from build123d import *

# Parameters (mm, degrees)
SKETCH1_R           = 12.5
SKETCH1_R_2         = 8
BOSS_EXTRUDE1_DEPTH = 2.5
SKETCH3_R           = 20
SKETCH3_R_2         = 8
BOSS_EXTRUDE3_DEPTH = 5
CHAMFER2_SIZE       = 1
SKETCH5_R           = 12.5
CUT_EXTRUDE1_DEPTH  = 10
CUT_EXTRUDE2_START  = -2
SKETCH6_R           = 2
CUT_EXTRUDE2_DEPTH  = 5


with BuildPart() as part:
    # Sketch1 → Boss-Extrude1 (new body)
    with BuildSketch(Plane.XY):
        Circle(SKETCH1_R)
        Circle(SKETCH1_R_2, mode=Mode.SUBTRACT)
    extrude(amount=BOSS_EXTRUDE1_DEPTH)

    # Sketch3 → Boss-Extrude3 (add)
    with BuildSketch(Plane(origin=(0, 0, 0), x_dir=(-1, 0, 0), z_dir=(0, 0, -1))):
        Circle(SKETCH3_R)
        Circle(SKETCH3_R_2, mode=Mode.SUBTRACT)
    extrude(amount=BOSS_EXTRUDE3_DEPTH)

    # Chamfer2
    chamfer2_edges = [part.edges().sort_by_distance(p)[0] for p in [
        (20, 0, 0),
        (20, 0, -5),
    ]]
    chamfer(chamfer2_edges, length=CHAMFER2_SIZE)

    # Sketch5 → Cut-Extrude1 (cut)
    with BuildSketch(Plane.XY):
        Circle(SKETCH5_R)
    extrude(amount=CUT_EXTRUDE1_DEPTH, mode=Mode.SUBTRACT)

    # Sketch6 → Cut-Extrude2 (cut)
    with BuildSketch(Plane(origin=(0, 0, -5), x_dir=(-1, 0, 0), z_dir=(0, 0, -1)).offset(CUT_EXTRUDE2_START)):
        with Locations((14, 0)):
            Circle(SKETCH6_R)
        with Locations((-14, 0)):
            Circle(SKETCH6_R)
    extrude(amount=-CUT_EXTRUDE2_DEPTH, mode=Mode.SUBTRACT)


solid = part.part
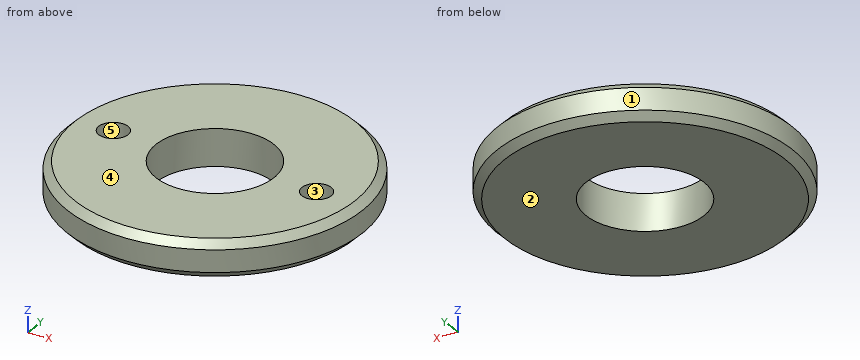
Can you work these out from the model? Positions are in its coordinate system, mm. Face numbers are marked on the shaded views. A direction names the side the tool comes from. Coordinates: 2 decimals unless noted, no trailing zeros. Loops run counter-clockwise (first coordinate to the right, second up) from the corner with the lowest first, then second, coordinate; pieces in that order, holes last. Notation, with made-up numbers: (39, 5) - (71, 5) arc R19 ccw to (71, 23) - close; hole circle Ø9 at (64, 21). An arc over 180 degrees is marked (long way). Put each result on its own line as item: value. Start each with the question number.
Item 1: If I drill on line 1 along Y through (x, z) = (0, -1.1); line 2 along Y through (x, z) = (-13.5, -1.4); line 3 along X through (y, z) = (-6, -1), over which ranges is the centre line in solid material (lowest first)?
Item 2: Suppose I cut it at B-B (x = 0). Please give me the cut outline in (y, z), and give its area (3 significant figures).
Item 3: Suppose I cut it at A-A (y = 0). Please give me the cut outline in (x, z).
Item 4: If we mould it in two halves opening along X, with no side actions, what happens to the marked faces 1, 2 and 3? For each: +X half, -X half, draft (parallel to the pull), parting line (faces both ways), or undercut.
Item 5: Which directions (+Z, -Z, +X, -X, +Y, -Y) give clear straight access to the entire face, cutting with the end or side of a thin tool? Please do the marked faces 4 and 5.
Item 6: Suppose I cut it at C-C (z = -1.75). Please give me the cut outline in (x, y).
Item 7: For pin 1 (1.5 mm diameter, centred on x = 15, z = -2.5, fed in from +Y); pin 2 (6 mm diameter, centred on x = -3, y = -0.5, fed in from +Z); pin 3 (1.2 mm diameter, centred on x = 15, y = -0.5, fed in from +Z); pin 4 (3 mm diameter, centred on y = -15.5, z = -4.5, fed in from +X), each with a flat end and sliding along its axis, tell me the tip position at first contact or that it passes through.
Here are the results:
1. line 1: -20 to -8, 8 to 20
1. line 2: -14.76 to -1.94, 1.94 to 14.76
1. line 3: -19.08 to -5.29, 5.29 to 19.08
2. outline: (-20, -4) - (-19, -5) - (-8, -5) - (-8, 0) - (-19, 0) - (-20, -1) - close; (8, -5) - (19, -5) - (20, -4) - (20, -1) - (19, 0) - (8, 0) - close
2. area: 118 mm²
3. outline: (-20, -4) - (-19, -5) - (-8, -5) - (-8, 0) - (-12, 0) - (-12, -3) - (-16, -3) - (-16, 0) - (-19, 0) - (-20, -1) - close; (8, -5) - (19, -5) - (20, -4) - (20, -1) - (19, 0) - (16, 0) - (16, -3) - (12, -3) - (12, 0) - (8, 0) - close
4. face 1: parting line
4. face 2: draft
4. face 3: undercut
5. face 4: +Z, +X, -X, +Y, -Y
5. face 5: +Z
6. outline: circle Ø40 at (0, 0); hole circle Ø4 at (-14, 0); hole circle Ø16 at (0, 0); hole circle Ø4 at (14, 0)
7. pin 1: y = 14.03
7. pin 2: through
7. pin 3: z = -3
7. pin 4: x = 14.2
